```python
from build123d import *

# Parameters (mm, degrees)
SKETCH2_R               = 2
BOSS_EXTRUDE1_DEPTH     = 28.866025404
CUT_EXTRUDE1_REACH      = 33.38
CUT_EXTRUDE1_END_RADIUS = 3.5
CHAMFER1_SIZE           = 0.5
CHAMFER1_SIZE2          = 0.866025404
FILLET1_R               = 0.5


with BuildPart() as part:
    # Sketch1 → Revolve1 (revolve)
    with BuildSketch(Plane(origin=(0, 0, 0), x_dir=(-1, 0, 0), z_dir=(0, 0, -1)), mode=Mode.PRIVATE) as revolve1_sk:
        with BuildLine():
            Line((14, 4), (14, 0))
            Line((14, 0), (19.5, 0))
            ThreePointArc((19.5, 0), (18.474873734, 2.474873734), (16, 3.5))
            Line((16, 3.5), (15, 3.5))
            Line((15, 3.5), (15, 4))
            Line((15, 4), (14, 4))
        make_face()
    revolve(revolve1_sk.sketch.rotate(Axis((-14, 0, 0), (-1, 0, 0)), 270), axis=Axis((-14, 0, 0), (-1, 0, 0)))

    # Sketch2 → Boss-Extrude1 (add)
    with BuildSketch(Plane(origin=(-14, 0, 0), x_dir=(0, 0, -1), z_dir=(1, 0, 0))):
        Circle(SKETCH2_R)
    extrude(amount=BOSS_EXTRUDE1_DEPTH)

    # Cut-Extrude1: up to this sphere (the profile starts inside it)
    cut_extrude1_end = Location((-16, 0, 0)) * Sphere(CUT_EXTRUDE1_END_RADIUS, mode=Mode.PRIVATE)
    # Sketch3 → Cut-Extrude1 (cut, up to the surface)
    with BuildSketch(Plane(origin=(-16, 0, 0), x_dir=(0, 0, -1), z_dir=(1, 0, 0)), mode=Mode.PRIVATE) as cut_extrude1_sk1:
        with BuildLine():
            Line((2.271345978, 1.959843731), (0.191997374, 0.590907157))
            Line((0.191997374, 0.590907157), (-0.685590254, 2.920610553))
            ThreePointArc((-0.685590254, 2.920610553), (-0.927050983, 2.853169549), (-1.162037644, 2.765803412))
            Line((-1.162037644, 2.765803412), (-0.502655651, 0.365200707))
            Line((-0.502655651, 0.365200707), (-2.989524738, 0.250483216))
            ThreePointArc((-2.989524738, 0.250483216), (-3, 0), (-2.989524738, -0.250483216))
            Line((-2.989524738, -0.250483216), (-0.502655651, -0.365200707))
            Line((-0.502655651, -0.365200707), (-1.162037644, -2.765803412))
            ThreePointArc((-1.162037644, -2.765803412), (-0.927050983, -2.853169549), (-0.685590254, -2.920610553))
            Line((-0.685590254, -2.920610553), (0.191997374, -0.590907157))
            Line((0.191997374, -0.590907157), (2.271345978, -1.959843731))
            ThreePointArc((2.271345978, -1.959843731), (2.427050983, -1.763355757), (2.565806659, -1.554553373))
            Line((2.565806659, -1.554553373), (0.621316554, 0))
            Line((0.621316554, 0), (2.565806659, 1.554553373))
            ThreePointArc((2.565806659, 1.554553373), (2.427050983, 1.763355757), (2.271345978, 1.959843731))
        make_face()
    cut_extrude1_tool1 = extrude(cut_extrude1_sk1.sketch, amount=-CUT_EXTRUDE1_REACH, mode=Mode.PRIVATE) & cut_extrude1_end
    add(cut_extrude1_tool1.solids().sort_by_distance((-16, 0, 0))[0], mode=Mode.SUBTRACT)

    # Chamfer1
    chamfer1_edges = [part.edges().sort_by_distance(p)[0] for p in [
        (14.866025404, 0, 2),
    ]]
    chamfer1_side = [part.faces().sort_by_distance(p)[0] for p in [
        (14.866025404, 0, 0),
    ]]
    chamfer(chamfer1_edges, length=CHAMFER1_SIZE, length2=CHAMFER1_SIZE2, reference=chamfer1_side[0])

    # Fillet1
    # the kernel refuses this fillet: 0.5 mm, written as the material it takes off along each edge
    with BuildSketch(Plane(origin=(-16, 0, -0.621316554), x_dir=(0, -0.6244406033134772, -0.7810722968672622), z_dir=(-1, 0, 0)), Plane(origin=(-16, -0.590907157, -0.191997374), x_dir=(0, -0.9358066560348443, 0.35251369125309573), z_dir=(-1, 0, 0)), Plane(origin=(-16, -0.365200707, 0.502655651), x_dir=(0, 0.04608028298555685, 0.9989377395613659), z_dir=(-1, 0, 0)), Plane(origin=(-16, 0.365200707, 0.502655651), x_dir=(0, 0.964285837131132, 0.2648637844408172), z_dir=(-1, 0, 0)), Plane(origin=(-16, 0.590907157, -0.191997374), x_dir=(0, 0.5498811392316572, -0.8352429183879951), z_dir=(-1, 0, 0))) as fillet1_piece_1:
        with BuildLine():
            CenterArc((FILLET1_R * 1.25083521591, -FILLET1_R), FILLET1_R, 90, 102.717718013)
            Line((FILLET1_R * 0.275368703333, -FILLET1_R * 1.22014786587), (0, 0))
            Line((0, 0), (FILLET1_R * 1.25083521591, 0))
        make_face()
    extrude(amount=5.007954817, mode=Mode.SUBTRACT)


solid = part.part
```
Verification items for the finished model (mm, model axes). A direction names the side the tool comes from. Coordinates: 2 decimals unless noted, no trailing zeros. Write each loop counter-clockwise with the first axis right and the second up, starting at its lowest first coordinate (ties: lowest second). Pieces come first, ordered by that corner, then holes. Notation, with made-up numbers: M 80.5,-21.75 L 138.5,-21.75 A21 cw 138.5,-2.75 Z; hole C 21.5,27 d8. An arc over 180 degrees is marked long. One line per item, written item: value.
Item 1: Section check A-A, the plane x = -1.5. Record the boundary of the cut face in (y, z).
Check sheet entries:
outline: C 0,0 d4
Item 2: Gauge pin test, flat ends, axial feed: pin 1 Ø4 at (x, z) = (11.5, -1.5) entering from +Y; pin 2 Ø1.5 at (y, z) = (1, -3) entering from +X; pin 3 Ø1 at (y, z) = (2.5, 0) entering from -X. Record the tip position at first contact, or that the pin passes through.
Check sheet entries:
pin 1: stops at y = 2
pin 2: stops at x = -14
pin 3: stops at x = -18.87
Item 3: Scan lines: line 1 along Y through (x, z) = (-4, -1.75); line 2 along X through (y, z) = (3, 2); line 3 along X through (y, z) = (-0.5, 0). Record each from-to range of solid material in increasing order.
Check sheet entries:
line 1: y = -0.97 to 0.97
line 2: x = -15 to -14
line 3: x = -16 to 14.87
Item 4: Access from +Z, -Z, +X, -X, +Y, -Y to the whole of each face (thin tool, end or side, straight path). Record for faces 1 (the flat face through (-17.259, 0.964, -1.828)), 2 (the flat face through (14.866, 0, 0)).
Check sheet entries:
face 1: -X
face 2: +Z, -Z, +X, +Y, -Y
Item 5: Mould release check, pull along Z, two halves, no side actions. Record for faces 3 (the flat face through (-17.26, 1.45, -1.5)), 4 (the cylindrical face through (0, -2, 0)), 5 (the flat face through (-14, -1, -2)): pulls with the +Z half, pulls with the -Z half, needs draft (parallel to the pull), parting line crosses it, or undercut.
Check sheet entries:
face 3: undercut
face 4: parting line crosses it
face 5: needs draft
